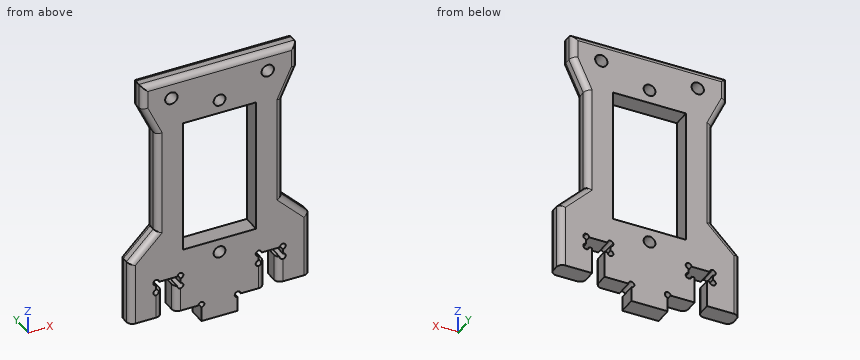
from build123d import *

# Parameters (mm, degrees)
F0_R     = 1.05
F0_R_2   = 1
F1_DEPTH = 3
F2_R     = 1


# Not quite as in the source:
# - a feature names something its author has since deleted; it is built from what else it names


with BuildPart() as f1:
    # F0 (on Front) → F1 (new body)
    with BuildSketch(Plane.XZ):
        with BuildLine():
            ThreePointArc((3.08, -22.97), (2.7264466094, -22.8235533906), (2.58, -22.47))
            Line((2.58, -22.47), (-2.58, -22.47))
            ThreePointArc((-2.58, -22.47), (-2.7264466094, -22.8235533906), (-3.08, -22.97))
            Line((-3.08, -22.97), (-3.08, -25.47))
            Line((-3.08, -25.47), (3.08, -25.47))
            Line((3.08, -25.47), (3.08, -22.97))
        make_face()
        Polygon((10.74, -6.94), (10.74, -11.5), (15.3, -11.5), align=None)
        Polygon((-15.3, -11.5), (-10.74, -11.5), (-10.74, -6.94), align=None)
        with BuildLine():
            Line((10.74, -11.5), (10.74, -15.61))
            ThreePointArc((10.74, -15.61), (11.24, -16.11), (10.74, -16.61))
            Line((10.74, -16.61), (10.74, -17.41))
            ThreePointArc((10.74, -17.41), (11.0935533906, -18.2635533906), (10.24, -17.91))
            Line((10.24, -17.91), (9.74, -17.91))
            Line((9.74, -17.91), (9.74, -22.47))
            Line((9.74, -22.47), (15.3, -22.47))
            Line((15.3, -22.47), (15.3, -11.5))
            Line((15.3, -11.5), (10.74, -11.5))
        make_face()
        with BuildLine():
            Line((-10.74, -15.61), (-10.74, -11.5))
            Line((-10.74, -11.5), (-15.3, -11.5))
            Line((-15.3, -11.5), (-15.3, -22.47))
            Line((-15.3, -22.47), (-9.74, -22.47))
            Line((-9.74, -22.47), (-9.74, -17.91))
            Line((-9.74, -17.91), (-10.24, -17.91))
            ThreePointArc((-10.24, -17.91), (-11.0935533906, -18.2635533906), (-10.74, -17.41))
            Line((-10.74, -17.41), (-10.74, -16.61))
            ThreePointArc((-10.74, -16.61), (-11.24, -16.11), (-10.74, -15.61))
        make_face()
        Polygon((6.18, -11.5), (10.74, -11.5), (10.74, -6.94), (10.74, 10.6763684678), (13.18, 15.9089653538), (13.18, 20.1089653538), (-13.18, 20.1089653538), (-13.18, 15.9089653538), (-10.74, 10.6763684678), (-10.74, -6.94), (-10.74, -11.5), (-6.18, -11.5), (-6.18, 11.5), (6.18, 11.5), align=None)
        with Locations((-8.18, 16.6589653538)):
            Circle(F0_R, mode=Mode.SUBTRACT)
        with Locations((0, 13.805)):
            Circle(F0_R_2, mode=Mode.SUBTRACT)
        with Locations((8.18, 16.6589653538)):
            Circle(F0_R, mode=Mode.SUBTRACT)
        with BuildLine():
            ThreePointArc((6.64, -16.61), (6.2864466094, -16.4635533906), (6.14, -16.11))
            Line((6.14, -16.11), (-6.14, -16.11))
            ThreePointArc((-6.14, -16.11), (-6.2864466094, -16.4635533906), (-6.64, -16.61))
            Line((-6.64, -16.61), (-6.64, -17.41))
            ThreePointArc((-6.64, -17.41), (-6.2864466094, -18.2635533906), (-7.14, -17.91))
            Line((-7.14, -17.91), (-7.64, -17.91))
            Line((-7.64, -17.91), (-7.64, -22.47))
            Line((-7.64, -22.47), (-3.58, -22.47))
            ThreePointArc((-3.58, -22.47), (-3.08, -21.97), (-2.58, -22.47))
            Line((-2.58, -22.47), (2.58, -22.47))
            ThreePointArc((2.58, -22.47), (3.08, -21.97), (3.58, -22.47))
            Line((3.58, -22.47), (7.64, -22.47))
            Line((7.64, -22.47), (7.64, -17.91))
            Line((7.64, -17.91), (7.14, -17.91))
            ThreePointArc((7.14, -17.91), (6.2864466094, -18.2635533906), (6.64, -17.41))
            Line((6.64, -17.41), (6.64, -16.61))
        make_face()
        with BuildLine():
            ThreePointArc((6.14, -16.11), (6.1501020514, -16.01), (6.18, -15.9140408206))
            Line((6.18, -15.9140408206), (6.18, -11.5))
            Line((6.18, -11.5), (-6.18, -11.5))
            Line((-6.18, -11.5), (-6.18, -15.9140408206))
            ThreePointArc((-6.18, -15.9140408206), (-6.1501020514, -16.01), (-6.14, -16.11))
            Line((-6.14, -16.11), (6.14, -16.11))
        make_face()
        with Locations((0, -13.805)):
            Circle(F0_R_2, mode=Mode.SUBTRACT)
        with BuildLine():
            Line((-6.18, -15.9140408206), (-6.18, -11.5))
            Line((-6.18, -11.5), (-10.74, -11.5))
            Line((-10.74, -11.5), (-10.74, -15.61))
            ThreePointArc((-10.74, -15.61), (-10.3864466094, -15.7564466094), (-10.24, -16.11))
            Line((-10.24, -16.11), (-7.14, -16.11))
            ThreePointArc((-7.14, -16.11), (-6.74, -15.6201020514), (-6.18, -15.9140408206))
        make_face()
        with BuildLine():
            Line((7.14, -16.11), (10.24, -16.11))
            ThreePointArc((10.24, -16.11), (10.3864466094, -15.7564466094), (10.74, -15.61))
            Line((10.74, -15.61), (10.74, -11.5))
            Line((10.74, -11.5), (6.18, -11.5))
            Line((6.18, -11.5), (6.18, -15.9140408206))
            ThreePointArc((6.18, -15.9140408206), (6.74, -15.6201020514), (7.14, -16.11))
        make_face()
    extrude(amount=F1_DEPTH)

    # F2
    f2_edges = [f1.edges().sort_by_distance(p)[0] for p in [
        (0, -3, 20.108965),
        (-13.18, -3, 18.008965),
        (-11.96, -3, 13.292667),
        (-10.74, -3, 1.868184),
        (-13.02, -3, -9.22),
        (-15.3, -3, -16.985),
        (15.3, -3, -16.985),
        (13.02, -3, -9.22),
        (10.74, -3, 1.868184),
        (11.96, -3, 13.292667),
        (13.18, -3, 18.008965),
        (7.64, -3, -20.19),
        (9.74, -3, -20.19),
        (-7.64, -3, -20.19),
        (-9.74, -3, -20.19),
        (0, 0, 20.108965),
        (13.18, 0, 18.008965),
        (11.96, 0, 13.292667),
        (-13.18, 0, 18.008965),
        (-11.96, 0, 13.292667),
        (-10.74, 0, 1.868184),
        (-13.02, 0, -9.22),
        (-15.3, 0, -16.985),
        (15.3, 0, -16.985),
        (13.02, 0, -9.22),
        (10.74, 0, 1.868184),
    ]]
    fillet(f2_edges, radius=F2_R)


solid = f1.part
Verification items for the finished model (mm, model axes). Round coordinates to 2 decimals unless told otherwise and drop trailing zeros. Loops run counter-clockwise (first coordinate to the right, second up) from the corner with the lowest first, then second, coordinate; pieces in that order, holes last. Notation, with made-up numbers: (-1.75, 37) - (41.25, 37) arc R12 ccw to (41.25, 53) - close; hole circle Ø8 at (-38.5, -34). An arc over 180 degrees is marked (long way). Use a Markdown table: item, result. Add a question column.
1. Thickness scan on probe 1 along Z at (x, y) = (0, -1.4) (3 decimals); probe 2 along X at (y, z) = (-1.6, 7); probe 3 along X at (y, z) = (-1.15, -20.5). Record the ranges inside material, lowest first. Write a range as [from, to].
2. Section check D-D, the plane x = -5. Record the boundary of the cut face in (y, z).
3. Gauge pin test, flat ends, axial feed: pin 1 (1 mm diameter, centred on y = -2, z = 11, fed in from -X); pin 2 (0.6 mm diameter, centred on x = -6.64, z = -17.91, fed in from -Y); pin 3 (0.9 mm diameter, centred on x = 8.5, y = -2, fed in from -Z); pin 4 (0.9 mm diameter, centred on y = -1, z = 1.5, fed in from -X). Record the tip position at first contact, or that the pin passes through.
4. Section check B-B, the plane z = 8. Record the boundary of the cut face in (x, y).
5. Section check A-A, the plane x = 8.18. Record the boundary of the cut face in (y, z).
6. Section check C-C, the plane x = 0. Record the boundary of the cut face in (y, z) (3 decimals).
Checks:
| question | item | result |
|---|---|---|
| 1 | probe 1 | z = [-25.47, -14.805], [-12.805, -11.5], [11.5, 12.805], [14.805, 20.109] |
| 1 | probe 2 | x = [-10.74, -6.18], [6.18, 10.74] |
| 1 | probe 3 | x = [-15.3, -9.74], [-7.64, 7.64], [9.74, 15.3] |
| 2 | outline | (-3, -22.47) - (0, -22.47) - (0, -11.5) - (-3, -11.5) - close; (-3, 11.5) - (0, 11.5) - (0, 19.11) arc R1 ccw to (-1, 20.11) - (-2, 20.11) arc R1 ccw to (-3, 19.11) - close |
| 3 | pin 1 | stops at x = -11.12 |
| 3 | pin 2 | passes through |
| 3 | pin 3 | stops at z = -16.11 |
| 3 | pin 4 | stops at x = -10.74 |
| 4 | outline | (-10.74, -2) arc R1 ccw to (-9.74, -3) - (-6.18, -3) - (-6.18, 0) - (-9.74, 0) arc R1 ccw to (-10.74, -1) - close; (6.18, -3) - (9.74, -3) arc R1 ccw to (10.74, -2) - (10.74, -1) arc R1 ccw to (9.74, 0) - (6.18, 0) - close |
| 5 | outline | (-3, -16.11) - (0, -16.11) - (0, 15.61) - (-3, 15.61) - close; (-3, 17.71) - (0, 17.71) - (0, 19.11) arc R1 ccw to (-1, 20.11) - (-2, 20.11) arc R1 ccw to (-3, 19.11) - close |
| 6 | outline | (-3, -25.47) - (0, -25.47) - (0, -14.805) - (-3, -14.805) - close; (-3, -12.805) - (0, -12.805) - (0, -11.5) - (-3, -11.5) - close; (-3, 11.5) - (0, 11.5) - (0, 12.805) - (-3, 12.805) - close; (-3, 14.805) - (0, 14.805) - (0, 19.109) arc R1 ccw to (-1, 20.109) - (-2, 20.109) arc R1 ccw to (-3, 19.109) - close |
